Answer from the drawing. Dimensions are ordinates in mm from the lowest x, y and z of the part. A direction names the side the tool comes from. Give positions to 0.01 mm unless a question says otherwise; leave off trailing zeros. Order: outer loops, then holes, each group sorted by start corner. A loop starts at its lowest first (then second) coordinate and runs counter-clockwise, first axis right, second up. Notation, with made-up numbers: (49, -34.75) - (70, -34.75) arc R21 cw to (70, -20.75) - close; hole circle Ø9 at (-4.75, -10). An arc over 180 degrees is marked (long way). Answer in a Markdown table with one row per item.
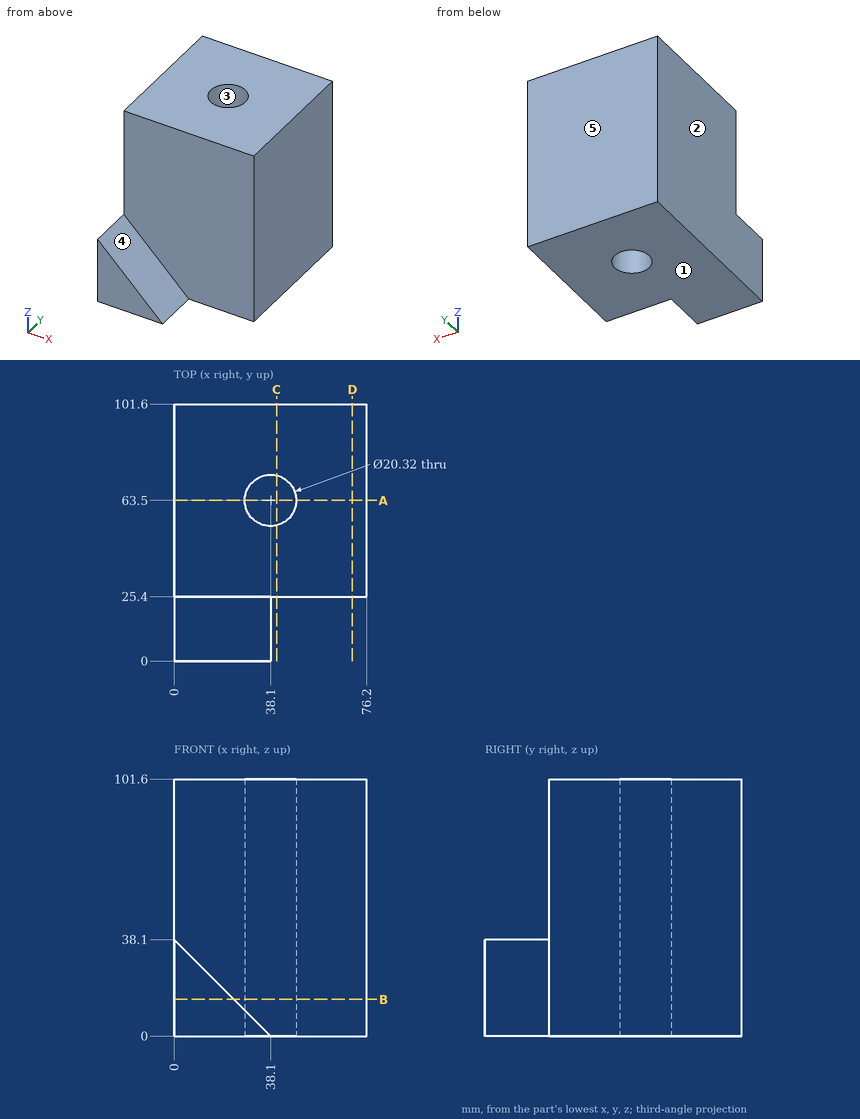
Item 1: Find section C-C on x = 40.5. Write down the section's boundary in (y, z), then the cut area to 3 significant figures.
Answer block:
| item | result |
|---|---|
| outline | (25.4, 0) - (53.63, 0) - (53.63, 101.6) - (25.4, 101.6) - close; (73.37, 0) - (101.6, 0) - (101.6, 101.6) - (73.37, 101.6) - close |
| area | 5,740 mm² |
Item 2: This flat-tipped pin is pushed along its axis until it touches: P1, Ø23, axis at x = 40, z = 65.5, coming from the -Y side. Where does it stop, or does it pass through?
Answer block:
| item | result |
|---|---|
| P1 | y = 25.4 |
Item 3: Which of the six approach directions +Z, -Z, +X, -X, +Y, -Y give full straight-line access (tool end or side, diameter ignored) to the marked faces 4 and 5?
Answer block:
| item | result |
|---|---|
| face 4 | +Z, +X, -Y |
| face 5 | +Z, -Z, +X, -X, +Y |
Item 4: Consider line 1 (X direction, y = 63, z = 41); line 2 (Y direction, x = 37.5, z = 64.5); line 3 (Y direction, x = 38.1, z = 80.5). Determine where each line is inside the solid, lowest interval first.
Answer block:
| item | result |
|---|---|
| line 1 | 0 to 27.95, 48.25 to 76.2 |
| line 2 | 25.4 to 53.36, 73.64 to 101.6 |
| line 3 | 25.4 to 53.34, 73.66 to 101.6 |
Item 5: Find section D-D on x = 70.5. Write down the section's boundary in (y, z), then the cut area to 3 significant figures.
Answer block:
| item | result |
|---|---|
| outline | (25.4, 0) - (101.6, 0) - (101.6, 101.6) - (25.4, 101.6) - close |
| area | 7,740 mm² |
Item 6: Find section A-A on y = 63.5. Write down the section's boundary in (x, z), then the cut area to 3 significant figures.
Answer block:
| item | result |
|---|---|
| outline | (0, 0) - (27.94, 0) - (27.94, 101.6) - (0, 101.6) - close; (48.26, 0) - (76.2, 0) - (76.2, 101.6) - (48.26, 101.6) - close |
| area | 5,680 mm² |
Item 7: Find section B-B on z = 14.5. Write down the section's boundary in (x, y), then the cut area to 3 significant figures.
Answer block:
| item | result |
|---|---|
| outline | (0, 0) - (23.6, 0) - (23.6, 25.4) - (76.2, 25.4) - (76.2, 101.6) - (0, 101.6) - close; hole circle Ø20.32 at (38.1, 63.5) |
| area | 6,080 mm² |
Item 8: Determine the mould class of the marked faces 1, 2 and 3 for opening direction X: pulls with the +X half, pulls with the -X half, needs draft (parallel to the pull), parting line crosses it, or undercut.
Answer block:
| item | result |
|---|---|
| face 1 | needs draft |
| face 2 | pulls with the -X half |
| face 3 | undercut |
